```python
from build123d import *

# Parameters (mm, degrees)
F0_R     = 19.05
F1_DEPTH = 63.5
F2_R     = 5.5626
F3_DEPTH = 20.6502


with BuildPart() as f1:
    # F0 (on Front) → F1 (new body)
    with BuildSketch(Plane.XZ):
        with BuildLine():
            Line((50.8, 28.575), (0, 28.575))
            ThreePointArc((0, 28.575), (-19.345366, -21.030631), (28.475608, 2.38125))
            ThreePointArc((28.475608, 2.38125), (30.957268, 9.623455), (37.967478, 12.7))
            Line((37.967478, 12.7), (50.8, 12.7))
            Line((50.8, 12.7), (50.8, 28.575))
        make_face()
        Circle(F0_R, mode=Mode.SUBTRACT)
    extrude(amount=F1_DEPTH)

    # F2 (on face) → F3 (join)
    with BuildSketch(Plane(origin=(0, 0, 12.7), x_dir=(1, 0, 0), z_dir=(0, 0, -1))):
        with BuildLine():
            ThreePointArc((50.8, 45.2374), (45.2374, 50.8), (50.8, 56.3626))
            Line((50.8, 56.3626), (50.8, 63.5))
            ThreePointArc((50.8, 63.5), (41.819744, 59.780256), (38.1, 50.8))
            Line((38.1, 50.8), (38.1, 12.7))
            ThreePointArc((38.1, 12.7), (41.819744, 3.719744), (50.8, 0))
            Line((50.8, 0), (50.8, 7.1374))
            ThreePointArc((50.8, 7.1374), (45.2374, 12.7), (50.8, 18.2626))
            Line((50.8, 18.2626), (50.8, 45.2374))
        make_face()
        with BuildLine():
            ThreePointArc((50.8, 56.3626), (54.733352, 54.733352), (56.3626, 50.8))
            ThreePointArc((56.3626, 50.8), (54.733352, 46.866648), (50.8, 45.2374))
            Line((50.8, 45.2374), (50.8, 18.2626))
            ThreePointArc((50.8, 18.2626), (54.733352, 16.633352), (56.3626, 12.7))
            ThreePointArc((56.3626, 12.7), (54.733352, 8.766648), (50.8, 7.1374))
            Line((50.8, 7.1374), (50.8, 0))
            ThreePointArc((50.8, 0), (54.058676, 0.425187), (57.099155, 1.672279))
            Line((57.099155, 1.672279), (90.449355, 20.722279))
            ThreePointArc((90.449355, 20.722279), (96.8502, 31.75), (90.449355, 42.777721))
            Line((90.449355, 42.777721), (57.099155, 61.827721))
            ThreePointArc((57.099155, 61.827721), (54.058676, 63.074813), (50.8, 63.5))
            Line((50.8, 63.5), (50.8, 56.3626))
        make_face()
        with Locations((84.1502, 31.75)):
            Circle(F2_R, mode=Mode.SUBTRACT)
    extrude(amount=-F3_DEPTH)


solid = f1.part
```
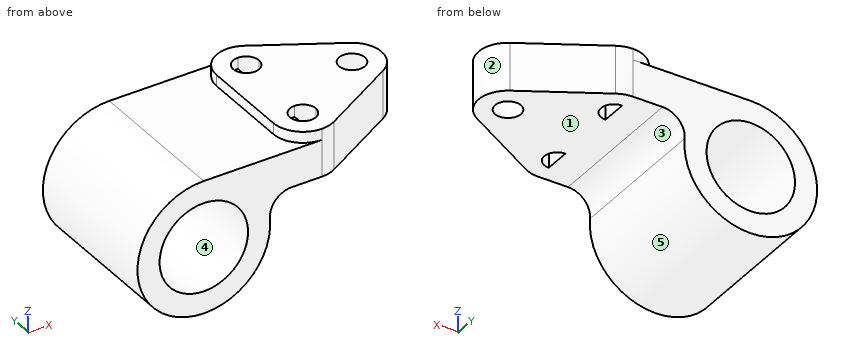
Here's how the part is built. I have some questions about the finished solid (model axes, mm). Face numbers are marked on the shaded views. A direction names the side the tool comes from. Coordinates: 2 decimals unless noted, no trailing zeros. Order: outer loops, then holes, each group sorted by start corner. A loop starts at its lowest first (then second) coordinate and runs counter-clockwise, first axis right, second up.
1) Will these pins go through, and if not, where does the flat tip stop? pin 1 (1.7 mm diameter, centred on x = 47.5, y = -10, fed in from +Z) (3 decimals); pin 2 (1.5 mm diameter, centred on y = -39, z = -9.5, fed in from -X); pin 3 (8 mm diameter, centred on x = 38, y = -13, fed in from -Z); pin 4 (6.5 mm diameter, centred on x = 84.15, y = -31.75, fed in from +Z).
2) We'd pull the mould along X, two halves only. Please class the marked faces 3, 4 and 5: +X half, -X half, draft (parallel to the pull), parting line (faces both ways), or undercut.
3) I need wall thicknesses on line 1 (Z direction, x = 1, y = -36) (1 decimal); line 2 (Z direction, x = 55.5, y = -27); line 3 (X direction, y = -58, z = -13). Which ranges of each line are inside material? Lowest first, please.
4) Imagine slicing it at A-A on y = -55. List the corners of the cut face in (x, z) for me (3 decimals).
5) Which directions (+Z, -Z, +X, -X, +Y, -Y) give clear straight access to the entire face, cutting with the end or side of a thin tool? Please do the marked faces 1 and 2.
6) Imagine slicing it at C-C on x = 11.5. List the corners of the cut face in (y, z) for me (3 decimals).
7) Imagine slicing it at B-B on z = 14. List the corners of the cut face in (x, y) for me.
8) Imagine slicing it at D-D on y = -39. List the corners of the cut face in (x, z) for me (3 decimals), and give its area (3 significant figures).
Response values:
1. pin 1: stops at z = 28.575
1. pin 2: stops at x = -27.2
1. pin 3: stops at z = 11.83
1. pin 4: passes through
2. face 3: +X half
2. face 4: undercut
2. face 5: parting line
3. line 1: z = -28.6 to -19, 19 to 28.6
3. line 2: z = 12.7 to 33.35
3. line 3: x = -25.45 to -13.92, 13.92 to 25.45
4. outline: (0, 28.575) arc R28.575 ccw (long way) to (28.476, 2.381) arc R9.525 cw to (37.967, 12.7) - (50.8, 12.7) - (50.8, 28.575) - (47.153, 28.575) - (47.153, 33.35) - (38.815, 33.35) - (38.815, 28.575) - close; (54.447, 12.7) - (69.052, 12.7) - (69.052, 33.35) - (54.447, 33.35) - close; hole circle Ø38.1 at (0, 0)
5. face 1: -Z, +X, +Y, -Y
5. face 2: +Z, -Z, +X
6. outline: (-63.5, -26.159) - (0, -26.159) - (0, -15.187) - (-63.5, -15.187) - close; (-63.5, 15.187) - (0, 15.187) - (0, 28.575) - (-63.5, 28.575) - close
7. outline: (-24.91, -63.5) - (-12.92, -63.5) - (-12.92, 0) - (-24.91, 0) - close; (12.92, -63.5) - (50.8, -63.5) arc R12.7 ccw to (57.1, -61.83) - (90.45, -42.78) arc R12.7 ccw to (90.45, -20.72) - (57.1, -1.67) arc R12.7 ccw to (50.8, 0) - (12.92, 0) - close; hole (50.8, -56.36) arc R5.56 ccw to (56.36, -50.8) arc R5.56 ccw to (50.8, -45.24) - close; hole (50.8, -18.26) arc R5.56 ccw to (56.36, -12.7) arc R5.56 ccw to (50.8, -7.14) - close; hole circle Ø11.13 at (84.15, -31.75)
8. outline: (0, 28.575) arc R28.575 ccw (long way) to (28.476, 2.381) arc R9.525 cw to (37.967, 12.7) - (94.577, 12.7) - (94.577, 33.35) - (38.1, 33.35) - (38.1, 28.575) - close; hole circle Ø38.1 at (0, 0)
8. area: 2,940 mm2
